CAD build for the part. Positions are in the model's coordinates, mm. A direction names the side the tool comes from. Round coordinates to 2 decimals unless told otherwise and drop trailing zeros. Order: outer loops, then holes, each group sorted by start corner. A loop starts at its lowest first (then second) coordinate and runs counter-clockwise, first axis right, second up. Notation, with made-up numbers: M 59,-4.75 L 84,-4.75 A6 cw 84,1.25 Z; hole C 52.5,-15 d8. An arc over 180 degrees is marked long. Put each result on its own line as item: value.
```python
from build123d import *

# Parameters (mm, degrees)
SKETCH1_W           = 82
SKETCH1_H           = 20
BOSS_EXTRUDE1_DEPTH = 1.6
SKETCH2_W           = 11.38
SKETCH2_H           = 11.38
BOSS_EXTRUDE2_DEPTH = 3.15
SKETCH2_3_W         = 13.5
SKETCH2_3_H         = 12.7
BOSS_EXTRUDE3_DEPTH = 6.53
SKETCH3_W           = 3.78
SKETCH3_H           = 3.78
BOSS_EXTRUDE4_DEPTH = 3.78
SKETCH5_W           = 5.190366076
SKETCH5_H           = 1.495
CUT_EXTRUDE1_DEPTH  = 10
SKETCH6_R           = 1.5
CUT_EXTRUDE2_DEPTH  = 50.848178502
FILLET1_R           = 3


with BuildPart() as part:
    # Sketch1 → Boss-Extrude1 (new body)
    with BuildSketch(Plane(origin=(0, 0, 0), x_dir=(1, 0, 0), z_dir=(0, 1, 0))):
        Rectangle(SKETCH1_W, SKETCH1_H)
    extrude(amount=BOSS_EXTRUDE1_DEPTH)

    # Sketch2 → Boss-Extrude2 (add)
    with BuildSketch(Plane(origin=(0, 1.6, 0), x_dir=(1, 0, 0), z_dir=(0, 1, 0))):
        with Locations((-8.47, 0)):
            Rectangle(SKETCH2_W, SKETCH2_H)
        with Locations((9.53, 0)):
            Rectangle(SKETCH2_W, SKETCH2_H)
        with Locations((27.53, 0)):
            Rectangle(SKETCH2_W, SKETCH2_H)
    extrude(amount=BOSS_EXTRUDE2_DEPTH)

    # Sketch2_3 → Boss-Extrude3 (add)
    with BuildSketch(Plane(origin=(0, 1.6, 0), x_dir=(1, 0, 0), z_dir=(0, 1, 0))):
        with Locations((-26.47, 0)):
            Rectangle(SKETCH2_3_W, SKETCH2_3_H)
    extrude(amount=BOSS_EXTRUDE3_DEPTH)

    # Sketch3 → Boss-Extrude4 (add)
    with BuildSketch(Plane(origin=(0, 4.75, 0), x_dir=(1, 0, 0), z_dir=(0, 1, 0))):
        with Locations((-8.47, 0)):
            Rectangle(SKETCH3_W, SKETCH3_H)
        with Locations((9.53, 0)):
            Rectangle(SKETCH3_W, SKETCH3_H)
        with Locations((27.53, 0)):
            Rectangle(SKETCH3_W, SKETCH3_H)
    extrude(amount=BOSS_EXTRUDE4_DEPTH)

    # Sketch4 → Revolve1 (revolve)
    with BuildSketch(Plane.XY):
        Polygon((-23.04, 8.13), (-23.04, 14.53), (-23.525, 14.53), (-23.525, 15.28), (-24.885, 15.28), (-24.885, 16.11), (-23.47, 16.11), (-23.47, 28.13), (-26.47, 28.13), (-26.47, 8.13), align=None)
    revolve(axis=Axis((-26.47, 8.13, 0), (0, 1, 0)))

    # Sketch5 → Cut-Extrude1 (cut)
    with BuildSketch(Plane(origin=(0, 28.13, 0), x_dir=(1, 0, 0), z_dir=(0, 1, 0))):
        with Locations((-26.47, 2.2525)):
            Rectangle(SKETCH5_W, SKETCH5_H)
    extrude(amount=-CUT_EXTRUDE1_DEPTH, mode=Mode.SUBTRACT)

    # Sketch6 → Cut-Extrude2 (cut, through all)
    with BuildSketch(Plane(origin=(0, 1.6, 0), x_dir=(1, 0, 0), z_dir=(0, 1, 0))):
        with Locations(Location((-38, 7, 0), (0, 0, 270))):
            Circle(SKETCH6_R)
        with Locations(Location((-38, -7, 0), (0, 0, 270))):
            Circle(SKETCH6_R)
        with Locations(Location((38, -7, 0), (0, 0, 270))):
            Circle(SKETCH6_R)
        with Locations(Location((38, 7, 0), (0, 0, 270))):
            Circle(SKETCH6_R)
    extrude(amount=-CUT_EXTRUDE2_DEPTH, mode=Mode.SUBTRACT)

    # Fillet1
    fillet1_edges = [part.edges().sort_by_distance(p)[0] for p in [
        (-41, 0.8, -10),
        (41, 0.8, -10),
        (41, 0.8, 10),
        (-41, 0.8, 10),
    ]]
    fillet(fillet1_edges, radius=FILLET1_R)


solid = part.part
```
Item 1: Tool access for faces 1 (the flat face through (10, 8.53, 0)), 2 (the flat face through (10, 7, -1.89)), 3 (the flat face through (-2.78, 3, 0)), 4 (the flat face through (-27, 5, 6.35)): list every direction of +Z, -Z, +X, -X, +Y, -Y with a clear straight run to the whole face (end or side of a thin tool).
Answers below:
face 1: +Z, -Z, +X, +Y
face 2: -Z, +X, +Y
face 3: +Z, -Z, +Y
face 4: +Z, +X, -X, +Y
Item 2: Band-saw the part on B-B on x = -26.47. Give the cut face in (y, z) (3 decimals).
Answers below:
outline: M 0,-10 L 1.6,-10 L 1.6,-6.35 L 8.13,-6.35 L 8.13,-3.43 L 14.53,-3.43 L 14.53,-2.945 L 15.28,-2.945 L 15.28,-1.585 L 16.11,-1.585 L 16.11,-3 L 18.13,-3 L 18.13,-1.505 L 28.13,-1.505 L 28.13,3 L 16.11,3 L 16.11,1.585 L 15.28,1.585 L 15.28,2.945 L 14.53,2.945 L 14.53,3.43 L 8.13,3.43 L 8.13,6.35 L 1.6,6.35 L 1.6,10 L 0,10 Z
Item 3: Band-saw the part on C-C on y = 25.75. Give the cut face in (x, z) (3 decimals), and give its area (3 significant figures).
Answers below:
outline: M -29.065,-1.505 L -23.875,-1.505 A3 ccw long Z
area: 22.8 mm²
Item 4: Pin check, flat tips, straight feed: P1, Ø4, axis at x = 27.5, z = -0.5, coming from the +Y side; P2, Ø5, axis at x = -29, y = 5.5, coming from the +Z side; P3, Ø6, axis at x = -10, z = -5, coming from the +Y side; P4, Ø1.8, axis at x = -38, z = 7, coming from the -Y side. Stop position of each tip, or through.
Answers below:
P1: y = 8.53
P2: z = 6.35
P3: y = 4.75
P4: through
Item 5: Mould opens along X. For faces 5 (the flat face through (-10.36, 7, 0)), 6 (the flat face through (33.22, 3, 0)), 7 (the flat face through (-1, 1, 10)) say: pulls with the +X half, pulls with the -X half, needs draft (parallel to the pull), parting line crosses it, or undercut.
Answers below:
face 5: undercut
face 6: pulls with the +X half
face 7: needs draft
Item 6: Band-saw the part on D-D on x = 0. Give the cut face in (y, z), and give its area (3 significant figures).
Answers below:
outline: M 0,-10 L 1.6,-10 L 1.6,10 L 0,10 Z
area: 32.0 mm²
Item 7: Probe line 1 along X through (y, z) = (0.4, 7); line 2 along Y through (x, z) = (-29, 1); line 3 along Y through (x, z) = (-34.5, 4.5). List the from-to ranges inside material, lowest first. Write a range as [from, to].
Answers below:
line 1: [-41, -39.5], [-36.5, 36.5], [39.5, 41]
line 2: [0, 15.28], [16.11, 28.13]
line 3: [0, 1.6]
Item 8: Band-saw the part on A-A on y = 6.25. Give the cut face in (x, z), and give its area (3 significant figures).
Answers below:
outline: M -33.22,-6.35 L -19.72,-6.35 L -19.72,6.35 L -33.22,6.35 Z; M -10.36,-1.89 L -6.58,-1.89 L -6.58,1.89 L -10.36,1.89 Z; M 7.64,-1.89 L 11.42,-1.89 L 11.42,1.89 L 7.64,1.89 Z; M 25.64,-1.89 L 29.42,-1.89 L 29.42,1.89 L 25.64,1.89 Z
area: 214 mm²
